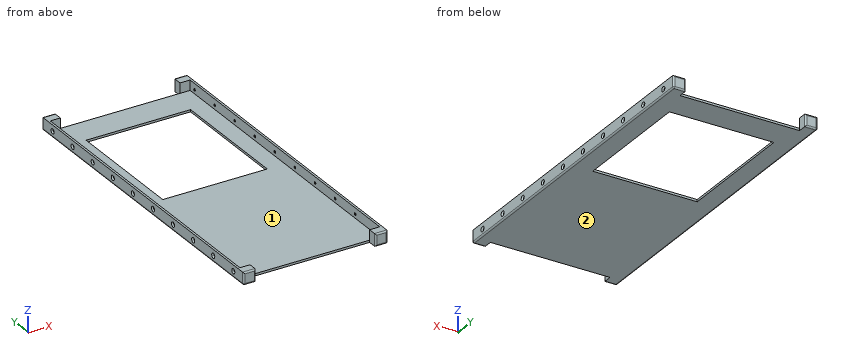
from build123d import *

# Parameters (mm, degrees)
BOSS_EXTRUDE1_DEPTH                           = 8.5
FILLET1_R                                     = 1
SKETCH2_W                                     = 83
SKETCH2_H                                     = 214
CUT_EXTRUDE1_DEPTH                            = 7
SKETCH3_W                                     = 97
SKETCH3_H                                     = 214
CUT_EXTRUDE2_DEPTH                            = 7
SKETCH6_W                                     = 36.25
SKETCH6_H                                     = 86.5
CUT_EXTRUDE3_DEPTH                            = 10
CSK_FOR_0_FLAT_HEAD_MACHINE_SCREW1_AT_2_COUNT = 2
CSK_FOR_0_FLAT_HEAD_MACHINE_SCREW1_AT_2_PITCH = 22.666666667
CSK_FOR_0_FLAT_HEAD_MACHINE_SCREW1_AT_3_COUNT = 2
CSK_FOR_0_FLAT_HEAD_MACHINE_SCREW1_AT_3_PITCH = 45.333333333
CSK_FOR_0_FLAT_HEAD_MACHINE_SCREW1_AT_4_COUNT = 2
CSK_FOR_0_FLAT_HEAD_MACHINE_SCREW1_AT_4_PITCH = 68
CSK_FOR_0_FLAT_HEAD_MACHINE_SCREW1_AT_5_COUNT = 2
CSK_FOR_0_FLAT_HEAD_MACHINE_SCREW1_AT_5_PITCH = 90.666666667
CSK_FOR_0_FLAT_HEAD_MACHINE_SCREW1_AT_6_COUNT = 2
CSK_FOR_0_FLAT_HEAD_MACHINE_SCREW1_AT_6_PITCH = 113.333333333
CSK_FOR_0_FLAT_HEAD_MACHINE_SCREW1_AT_7_COUNT = 2
CSK_FOR_0_FLAT_HEAD_MACHINE_SCREW1_AT_7_PITCH = 136
CSK_FOR_0_FLAT_HEAD_MACHINE_SCREW1_AT_8_COUNT = 2
CSK_FOR_0_FLAT_HEAD_MACHINE_SCREW1_AT_8_PITCH = 158.666666667
CSK_FOR_0_FLAT_HEAD_MACHINE_SCREW1_AT_9_COUNT = 2
CSK_FOR_0_FLAT_HEAD_MACHINE_SCREW1_AT_9_PITCH = 181.333333333
CSK_FOR_0_FLAT_HEAD_MACHINE_SCREW1_AT_1_COUNT = 2
CSK_FOR_0_FLAT_HEAD_MACHINE_SCREW1_AT_1_PITCH = 204


with BuildPart() as part:
    # Sketch1 → Boss-Extrude1 (new body)
    with BuildSketch(Plane.XY):
        Polygon((-41.5, -107), (41.5, -107), (41.5, -113.5), (50, -113.5), (50, -107), (50, 107), (50, 113.5), (41.5, 113.5), (41.5, 107), (-41.5, 107), (-41.5, 113.5), (-50, 113.5), (-50, 107), (-50, -107), (-50, -113.5), (-41.5, -113.5), align=None)
    extrude(amount=BOSS_EXTRUDE1_DEPTH)

    # Fillet1
    fillet1_edges = [part.edges().sort_by_distance(p)[0] for p in [
        (50, 0, 0),
        (45.75, -113.5, 0),
        (-45.75, -113.5, 0),
        (-50, 0, 0),
        (-45.75, 113.5, 0),
        (-45.75, 113.5, 8.5),
        (45.75, 113.5, 0),
        (50, -113.5, 4.25),
        (41.5, -113.5, 4.25),
        (-41.5, -113.5, 4.25),
        (-50, -113.5, 4.25),
        (-50, 113.5, 4.25),
        (-41.5, 113.5, 4.25),
        (41.5, 113.5, 4.25),
        (50, 113.5, 4.25),
        (-45.75, -113.5, 8.5),
        (45.75, -113.5, 8.5),
        (45.75, 113.5, 8.5),
    ]]
    fillet(fillet1_edges, radius=FILLET1_R)

    # Sketch2 → Cut-Extrude1 (cut)
    with BuildSketch(Plane.XY.offset(8.5)):
        Rectangle(SKETCH2_W, SKETCH2_H)
    extrude(amount=-CUT_EXTRUDE1_DEPTH, mode=Mode.SUBTRACT)

    # Sketch3 → Cut-Extrude2 (cut)
    with BuildSketch(Plane.XY.offset(8.5)):
        Rectangle(SKETCH3_W, SKETCH3_H)
    extrude(amount=-CUT_EXTRUDE2_DEPTH, mode=Mode.SUBTRACT)

    # Sketch6 → Cut-Extrude3 (cut)
    with BuildSketch(Plane(origin=(0, 0, 0), x_dir=(-1, 0, 0), z_dir=(0, 0, -1))):
        with Locations((-18.125, 43.25)):
            Rectangle(SKETCH6_W, SKETCH6_H)
        with Locations((18.125, 43.25)):
            Rectangle(SKETCH6_W, SKETCH6_H)
    extrude(amount=-CUT_EXTRUDE3_DEPTH, mode=Mode.SUBTRACT)

    # Sketch7 → CSK for #0 Flat Head Machine Screw1 (revolve, cut)
    with BuildSketch(Plane(origin=(50, 102, 4.25), x_dir=(0, 0, -1), z_dir=(0, 1, 0))):
        Polygon((0, 0), (0, 3.83616509), (0.889, 3.302), (0.889, 0.969878135), (1.7321022, 0), align=None)
    csk_for_0_flat_head_machine_screw1 = revolve(axis=Axis((56.35, 102, 4.25), (-1, 0, 0)), mode=Mode.SUBTRACT)

    # CSK for #0 Flat Head Machine Screw1 at 2: CSK for #0 Flat Head Machine Screw1 ×2
    with Locations(*[(0, -i * CSK_FOR_0_FLAT_HEAD_MACHINE_SCREW1_AT_2_PITCH, 0) for i in range(1, CSK_FOR_0_FLAT_HEAD_MACHINE_SCREW1_AT_2_COUNT)]):
        add(csk_for_0_flat_head_machine_screw1, mode=Mode.SUBTRACT)

    # CSK for #0 Flat Head Machine Screw1 at 3: CSK for #0 Flat Head Machine Screw1 ×2
    with Locations(*[(0, -i * CSK_FOR_0_FLAT_HEAD_MACHINE_SCREW1_AT_3_PITCH, 0) for i in range(1, CSK_FOR_0_FLAT_HEAD_MACHINE_SCREW1_AT_3_COUNT)]):
        add(csk_for_0_flat_head_machine_screw1, mode=Mode.SUBTRACT)

    # CSK for #0 Flat Head Machine Screw1 at 4: CSK for #0 Flat Head Machine Screw1 ×2
    with Locations(*[(0, -i * CSK_FOR_0_FLAT_HEAD_MACHINE_SCREW1_AT_4_PITCH, 0) for i in range(1, CSK_FOR_0_FLAT_HEAD_MACHINE_SCREW1_AT_4_COUNT)]):
        add(csk_for_0_flat_head_machine_screw1, mode=Mode.SUBTRACT)

    # CSK for #0 Flat Head Machine Screw1 at 5: CSK for #0 Flat Head Machine Screw1 ×2
    with Locations(*[(0, -i * CSK_FOR_0_FLAT_HEAD_MACHINE_SCREW1_AT_5_PITCH, 0) for i in range(1, CSK_FOR_0_FLAT_HEAD_MACHINE_SCREW1_AT_5_COUNT)]):
        add(csk_for_0_flat_head_machine_screw1, mode=Mode.SUBTRACT)

    # CSK for #0 Flat Head Machine Screw1 at 6: CSK for #0 Flat Head Machine Screw1 ×2
    with Locations(*[(0, -i * CSK_FOR_0_FLAT_HEAD_MACHINE_SCREW1_AT_6_PITCH, 0) for i in range(1, CSK_FOR_0_FLAT_HEAD_MACHINE_SCREW1_AT_6_COUNT)]):
        add(csk_for_0_flat_head_machine_screw1, mode=Mode.SUBTRACT)

    # CSK for #0 Flat Head Machine Screw1 at 7: CSK for #0 Flat Head Machine Screw1 ×2
    with Locations(*[(0, -i * CSK_FOR_0_FLAT_HEAD_MACHINE_SCREW1_AT_7_PITCH, 0) for i in range(1, CSK_FOR_0_FLAT_HEAD_MACHINE_SCREW1_AT_7_COUNT)]):
        add(csk_for_0_flat_head_machine_screw1, mode=Mode.SUBTRACT)

    # CSK for #0 Flat Head Machine Screw1 at 8: CSK for #0 Flat Head Machine Screw1 ×2
    with Locations(*[(0, -i * CSK_FOR_0_FLAT_HEAD_MACHINE_SCREW1_AT_8_PITCH, 0) for i in range(1, CSK_FOR_0_FLAT_HEAD_MACHINE_SCREW1_AT_8_COUNT)]):
        add(csk_for_0_flat_head_machine_screw1, mode=Mode.SUBTRACT)

    # CSK for #0 Flat Head Machine Screw1 at 9: CSK for #0 Flat Head Machine Screw1 ×2
    with Locations(*[(0, -i * CSK_FOR_0_FLAT_HEAD_MACHINE_SCREW1_AT_9_PITCH, 0) for i in range(1, CSK_FOR_0_FLAT_HEAD_MACHINE_SCREW1_AT_9_COUNT)]):
        add(csk_for_0_flat_head_machine_screw1, mode=Mode.SUBTRACT)

    # CSK for #0 Flat Head Machine Screw1 at 1: CSK for #0 Flat Head Machine Screw1 ×2
    with Locations(*[(0, -i * CSK_FOR_0_FLAT_HEAD_MACHINE_SCREW1_AT_1_PITCH, 0) for i in range(1, CSK_FOR_0_FLAT_HEAD_MACHINE_SCREW1_AT_1_COUNT)]):
        add(csk_for_0_flat_head_machine_screw1, mode=Mode.SUBTRACT)

    # Mirror1: CSK for #0 Flat Head Machine Screw1 across plane
    add(csk_for_0_flat_head_machine_screw1.mirror(Plane(origin=(0, 0, 0), x_dir=(0, 0, 1), z_dir=(1, 0, 0))), mode=Mode.SUBTRACT)

    # Mirror1 copy 1 sketch → Mirror1 copy 1 (revolve, cut)
    with BuildSketch(Plane(origin=(-50, 79.333333333, 4.25), x_dir=(0, 0, -1), z_dir=(0, 1, 0))):
        Polygon((0, 0), (0, -3.83616509), (0.889, -3.302), (0.889, -0.969878135), (1.7321022, 0), align=None)
    revolve(axis=Axis((-56.35, 79.333333333, 4.25), (-1, 0, 0)), mode=Mode.SUBTRACT)

    # Mirror1 copy 2 sketch → Mirror1 copy 2 (revolve, cut)
    with BuildSketch(Plane(origin=(-50, 56.666666667, 4.25), x_dir=(0, 0, -1), z_dir=(0, 1, 0))):
        Polygon((0, 0), (0, -3.83616509), (0.889, -3.302), (0.889, -0.969878135), (1.7321022, 0), align=None)
    revolve(axis=Axis((-56.35, 56.666666667, 4.25), (-1, 0, 0)), mode=Mode.SUBTRACT)

    # Mirror1 copy 3 sketch → Mirror1 copy 3 (revolve, cut)
    with BuildSketch(Plane(origin=(-50, 34, 4.25), x_dir=(0, 0, -1), z_dir=(0, 1, 0))):
        Polygon((0, 0), (0, -3.83616509), (0.889, -3.302), (0.889, -0.969878135), (1.7321022, 0), align=None)
    revolve(axis=Axis((-56.35, 34, 4.25), (-1, 0, 0)), mode=Mode.SUBTRACT)

    # Mirror1 copy 4 sketch → Mirror1 copy 4 (revolve, cut)
    with BuildSketch(Plane(origin=(-50, 11.333333333, 4.25), x_dir=(0, 0, -1), z_dir=(0, 1, 0))):
        Polygon((0, 0), (0, -3.83616509), (0.889, -3.302), (0.889, -0.969878135), (1.7321022, 0), align=None)
    revolve(axis=Axis((-56.35, 11.333333333, 4.25), (-1, 0, 0)), mode=Mode.SUBTRACT)

    # Mirror1 copy 5 sketch → Mirror1 copy 5 (revolve, cut)
    with BuildSketch(Plane(origin=(-50, -11.333333333, 4.25), x_dir=(0, 0, -1), z_dir=(0, 1, 0))):
        Polygon((0, 0), (0, -3.83616509), (0.889, -3.302), (0.889, -0.969878135), (1.7321022, 0), align=None)
    revolve(axis=Axis((-56.35, -11.333333333, 4.25), (-1, 0, 0)), mode=Mode.SUBTRACT)

    # Mirror1 copy 6 sketch → Mirror1 copy 6 (revolve, cut)
    with BuildSketch(Plane(origin=(-50, -34, 4.25), x_dir=(0, 0, -1), z_dir=(0, 1, 0))):
        Polygon((0, 0), (0, -3.83616509), (0.889, -3.302), (0.889, -0.969878135), (1.7321022, 0), align=None)
    revolve(axis=Axis((-56.35, -34, 4.25), (-1, 0, 0)), mode=Mode.SUBTRACT)

    # Mirror1 copy 7 sketch → Mirror1 copy 7 (revolve, cut)
    with BuildSketch(Plane(origin=(-50, -56.666666667, 4.25), x_dir=(0, 0, -1), z_dir=(0, 1, 0))):
        Polygon((0, 0), (0, -3.83616509), (0.889, -3.302), (0.889, -0.969878135), (1.7321022, 0), align=None)
    revolve(axis=Axis((-56.35, -56.666666667, 4.25), (-1, 0, 0)), mode=Mode.SUBTRACT)

    # Mirror1 copy 8 sketch → Mirror1 copy 8 (revolve, cut)
    with BuildSketch(Plane(origin=(-50, -79.333333333, 4.25), x_dir=(0, 0, -1), z_dir=(0, 1, 0))):
        Polygon((0, 0), (0, -3.83616509), (0.889, -3.302), (0.889, -0.969878135), (1.7321022, 0), align=None)
    revolve(axis=Axis((-56.35, -79.333333333, 4.25), (-1, 0, 0)), mode=Mode.SUBTRACT)

    # Mirror1 copy 9 sketch → Mirror1 copy 9 (revolve, cut)
    with BuildSketch(Plane(origin=(-50, -102, 4.25), x_dir=(0, 0, -1), z_dir=(0, 1, 0))):
        Polygon((0, 0), (0, -3.83616509), (0.889, -3.302), (0.889, -0.969878135), (1.7321022, 0), align=None)
    revolve(axis=Axis((-56.35, -102, 4.25), (-1, 0, 0)), mode=Mode.SUBTRACT)


solid = part.part
Check sheet for the modelled part. Datum: model origin and axes. Units: mm. Face numbers are marked on the shaded views. Round coordinates to 2 decimals unless told otherwise and drop trailing zeros. Write each loop counter-clockwise with the first axis right and the second up, starting at its lowest first coordinate (ties: lowest second). Pieces come first, ordered by that corner, then holes. Notation, with made-up numbers: (-30, 23) - (14, 23) arc R7 ccw to (14, 28) - close; hole circle Ø4 at (16, -1). An arc over 180 degrees is marked (long way). Return JSON: item names as keys, results as strings.
Q1. Depth check by flat-ended pin: P1, Ø1.6, axis at x = 8.5, z = 1, coming from the +Y side; P2, Ø2, axis at y = 56.67, z = 4.25, coming from the -X side; P3, Ø0.8, axis at x = -4, z = 0.5, coming from the -Y side. Enter the tip coordinate at first touch or a pass-through.
Returned:
{"P1": "stops at y = 107", "P2": "stops at x = -49.16", "P3": "stops at y = -107"}
Q2. Draft check along X on the marked faces 1 and 2. Enter one of: released by +X, released by -X, zero draft, split by the parting line, or undercut.
Returned:
{"face 1": "undercut", "face 2": "zero draft"}
Q3. Cross-section at B-B (x = 21). Record the boundary of the cut face in (y, z), then the cut area to 3 significant figures.
Returned:
{"outline": "(-107, 0) - (0, 0) - (0, 1.5) - (-107, 1.5) - close; (86.5, 0) - (107, 0) - (107, 1.5) - (86.5, 1.5) - close", "area": "191 mm²"}
Q4. Scan lines: L1, parallel to Y at x = 44, z = 3; L2, parallel to X at y = 19, z = 7; L3, parallel to X at y = 63.5, z = 1.25. Record each from-to range of solid material in increasing order. Write a range as from..to.
Returned:
{"L1": "y = -113.5..-107, 107..113.5", "L2": "x = -50..-48.5, 48.5..50", "L3": "x = -50..-36.25, 36.25..50"}
Q5. Cross-section at A-A (y = 84.5). Record the boundary of the cut face in (x, z), then the cut area to 3 significant figures.
Returned:
{"outline": "(-50, 1) arc R1 ccw to (-49, 0) - (-36.25, 0) - (-36.25, 1.5) - (-48.5, 1.5) - (-48.5, 8.5) - (-50, 8.5) - close; (36.25, 0) - (49, 0) arc R1 ccw to (50, 1) - (50, 8.5) - (48.5, 8.5) - (48.5, 1.5) - (36.25, 1.5) - close", "area": "61.8 mm²"}
Q6. Cross-section at C-C (y = -72.5). Record the boundary of the cut face in (x, z), then the cut area to 3 significant figures.
Returned:
{"outline": "(-50, 1) arc R1 ccw to (-49, 0) - (49, 0) arc R1 ccw to (50, 1) - (50, 8.5) - (48.5, 8.5) - (48.5, 1.5) - (-48.5, 1.5) - (-48.5, 8.5) - (-50, 8.5) - close", "area": "171 mm²"}
